```python
from build123d import *

# Parameters (mm, degrees)
SKETCH1_W           = 130
SKETCH1_H           = 130
SKETCH1_W_2         = 5
BOSS_EXTRUDE1_DEPTH = 3
SKETCH7_R           = 1.5
CUT_EXTRUDE3_DEPTH  = 3
SKETCH8_W           = 10
SKETCH8_H           = 5
BOSS_EXTRUDE5_DEPTH = 12
SKETCH9_R           = 1.5
CUT_EXTRUDE4_DEPTH  = 9
SKETCH10_W          = 5
SKETCH10_H          = 90
BOSS_EXTRUDE6_DEPTH = 12
SKETCH12_R          = 1.5
BOSS_EXTRUDE7_DEPTH = 3
CUT_EXTRUDE5_DEPTH  = 10


with BuildPart() as part:
    # Sketch1 → Boss-Extrude1 (new body)
    with BuildSketch(Plane(origin=(0, 0, 0), x_dir=(1, 0, 0), z_dir=(0, 1, 0))):
        Rectangle(SKETCH1_W, SKETCH1_H)
        with Locations((-67.5, 0)):
            Rectangle(SKETCH1_W_2, SKETCH1_H)
    extrude(amount=BOSS_EXTRUDE1_DEPTH)

    # Sketch7 → Cut-Extrude3 (cut)
    with BuildSketch(Plane(origin=(0, 3, 0), x_dir=(1, 0, 0), z_dir=(0, 1, 0))):
        with Locations(Location((-47.5, -62.5, 0), (0, 0, 270))):
            Circle(SKETCH7_R)
        with Locations(Location((-62.5, -62.5, 0), (0, 0, 270))):
            Circle(SKETCH7_R)
        with Locations(Location((-62.5, 22.5, 0), (0, 0, 270))):
            Circle(SKETCH7_R)
        with Locations(Location((-47.5, 22.5, 0), (0, 0, 90))):
            Circle(SKETCH7_R)
        with Locations(Location((-27.5, 22.5, 0), (0, 0, 270))):
            Circle(SKETCH7_R)
        with Locations(Location((-12.5, 22.5, 0), (0, 0, 90))):
            Circle(SKETCH7_R)
        with Locations(Location((-27.5, -62.5, 0), (0, 0, 90))):
            Circle(SKETCH7_R)
        with Locations(Location((-12.5, -62.5, 0), (0, 0, 270))):
            Circle(SKETCH7_R)
    extrude(amount=-CUT_EXTRUDE3_DEPTH, mode=Mode.SUBTRACT)

    # Sketch8 → Boss-Extrude5 (add)
    with BuildSketch(Plane(origin=(0, 3, 0), x_dir=(1, 0, 0), z_dir=(0, 1, 0))):
        Polygon((60, -65), (65, -65), (65, 40), (60, 40), (60, -29), (6, -29), (6, 60), (11, 60), (11, 65), (1, 65), (1, -34), (60, -34), align=None)
        with Locations((60, 62.5)):
            Rectangle(SKETCH8_W, SKETCH8_H)
    extrude(amount=BOSS_EXTRUDE5_DEPTH)

    # Sketch9 → Cut-Extrude4 (cut)
    with BuildSketch(Plane(origin=(0, 3, 0), x_dir=(1, 0, 0), z_dir=(0, 1, 0))):
        with Locations(Location((-63.5, 59, 0), (0, 0, 270))):
            Circle(SKETCH9_R)
        with Locations(Location((-63.5, 36, 0), (0, 0, 270))):
            Circle(SKETCH9_R)
        with Locations(Location((-5.5, 36, 0), (0, 0, 270))):
            Circle(SKETCH9_R)
        with Locations(Location((-5.5, 59, 0), (0, 0, 270))):
            Circle(SKETCH9_R)
    extrude(amount=-CUT_EXTRUDE4_DEPTH, mode=Mode.SUBTRACT)

    # Sketch10 → Boss-Extrude6 (add)
    with BuildSketch(Plane(origin=(0, 3, 0), x_dir=(1, 0, 0), z_dir=(0, 1, 0))):
        Polygon((-70, 30), (-70, 25), (-65, 25), (-14, 25), (-14, 30), align=None)
        with Locations((-67.5, -20)):
            Rectangle(SKETCH10_W, SKETCH10_H)
    extrude(amount=BOSS_EXTRUDE6_DEPTH)

    # Sketch12 → Boss-Extrude7 (add)
    with BuildSketch(Plane(origin=(0, 0, 0), x_dir=(1, 0, 0), z_dir=(0, 1, 0))):
        Polygon((65, -65), (60, -65), (-65, -65), (-70, -65), (-70, -70), (65, -70), align=None)
        with Locations(Location((60, -67.5, 0), (0, 0, 270))):
            Circle(SKETCH12_R, mode=Mode.SUBTRACT)
    extrude(amount=BOSS_EXTRUDE7_DEPTH)

    # Sketch13 → Cut-Extrude5 (cut)
    with BuildSketch(Plane(origin=(0, 15, 0), x_dir=(1, 0, 0), z_dir=(0, 1, 0))):
        with BuildLine():
            ThreePointArc((61.5, 62.5), (61.060660172, 63.560660172), (60, 64))
            Line((60, 64), (60, 61))
            ThreePointArc((60, 61), (61.060660172, 61.439339828), (61.5, 62.5))
        make_face()
        with BuildLine():
            Line((60, 61), (60, 64))
            ThreePointArc((60, 64), (58.5, 62.5), (60, 61))
        make_face()
    extrude(amount=-CUT_EXTRUDE5_DEPTH, mode=Mode.SUBTRACT)


solid = part.part
```
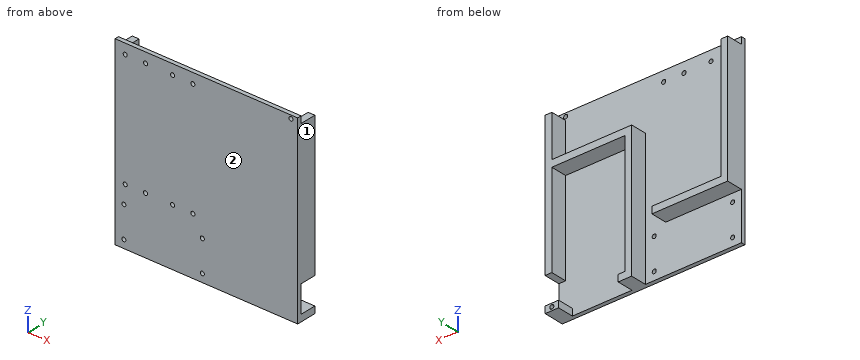
Could you check a few things on this model? Use its own coordinates, in mm. Face numbers are marked on the shaded views. Round coordinates to 2 decimals unless told otherwise and drop trailing zeros. Loops run counter-clockwise (first coordinate to the right, second up) from the corner with the lowest first, then second, coordinate; pieces in that order, holes last.
Q1. I want a section at D-D (z = 59). Write out the boundary of the cut face in (x, y), and give its area (3 significant figures).
Q2. I want a section at B-B (z = 4). Write out the boundary of the cut face in (x, y), and give its area (3 significant figures).
Q3. I want a section at A-A (y = 11.5). Write out the boundary of the cut face in (x, z).
Q4. Please list where these lines run through material, in increasing order: L1, parallel to X at y = 0.9, z = -59; L2, parallel to X at y = 0.8, z = -22.5; L3, parallel to X at y = 13, z = 25.
Q5. I want a section at C-C (x = 9). Write out the boundary of the cut face in (y, z), and give its area (3 significant figures).
Q6. Thinking about a two-plate mould opening in Y: for the marked faces 1 and 2, which applies, pulls with the +Y half, pulls with the -Y half, needs draft (parallel to the pull), parting line crosses it, or undercut?
Q7. For P1, Ø1.8, axis at x = -63.5, z = -36, coming from the -Y side; P2, Ø0.9, axis at x = 60.5, z = -62.5, coming from the +Y side; P3, Ø6, axis at x = 30.5, z = 45, coming from the +Y side; P4, Ø1.5, axis at x = -20.5, y = 11, coming from the -Z side, each with a flat end and sliding along its axis, tell me the tip position at first contact or that it passes through.
Answer below:
1. outline: (-70, 0) - (65, 0) - (65, 15) - (60, 15) - (60, 3) - (-65, 3) - (-65, 15) - (-70, 15) - close
1. area: 525 mm2
2. outline: (-70, 0) - (65, 0) - (65, 15) - (60, 15) - (60, 3) - (6, 3) - (6, 15) - (1, 15) - (1, 3) - (-65, 3) - (-65, 15) - (-70, 15) - close
2. area: 585 mm2
3. outline: (-70, -30) - (-14, -30) - (-14, -25) - (-65, -25) - (-65, 65) - (-70, 65) - close; (1, -65) - (11, -65) - (11, -60) - (6, -60) - (6, 29) - (60, 29) - (60, -40) - (65, -40) - (65, 65) - (60, 65) - (60, 34) - (1, 34) - close; (55, -65) - (65, -65) - (65, -60) - (55, -60) - close; hole circle Ø3 at (60, -62.5)
4. L1: x = -70 to -65, -62 to -7, -4 to 65
4. L2: x = -70 to -64, -61 to -49, -46 to -29, -26 to -14, -11 to 65
4. L3: x = -70 to -65, 1 to 6, 60 to 65
5. outline: (0, -65) - (15, -65) - (15, -60) - (3, -60) - (3, 29) - (15, 29) - (15, 34) - (3, 34) - (3, 70) - (0, 70) - close
5. area: 525 mm2
6. face 1: needs draft
6. face 2: pulls with the -Y half
7. P1: passes through
7. P2: stops at y = 5
7. P3: stops at y = 3
7. P4: stops at z = -30
